Verification items for the finished model (mm, model axes). Give positions to 0.01 mm unless a question says otherwise; leave off trailing zeros. Order: outer loops, then holes, each group sorted by start corner. A loop starts at its lowest first (then second) coordinate and runs counter-clockwise, first axis right, second up.
(1) Sectioned sample at B-B on x = 30. Record the cut outline in (y, z), plus the area to 3 significant figures.
(2) Scan lines: L1, parallel to X at y = -48.5, z = 2.75; L2, parallel to X at y = 82, z = 0.8; L3, parallel to Y at x = 93, z = 2.6. Record each from-to range of solid material in increasing order.
(3) Sectioned sample at A-A on y = 37. Record the cut outline in (x, z), plus the area to 3 significant figures.
(4) Gauge pin test, flat ends, axial feed: pin 1 (0.9 mm diameter, centred on x = 106, z = 1, fed in from +Y); pin 2 (0.9 mm diameter, centred on y = -102, z = 1, fed in from -X); pin 3 (0.9 mm diameter, centred on x = -106.5, z = 1, fed in from -Y). Record the tip position at first contact, or that the pin passes through.
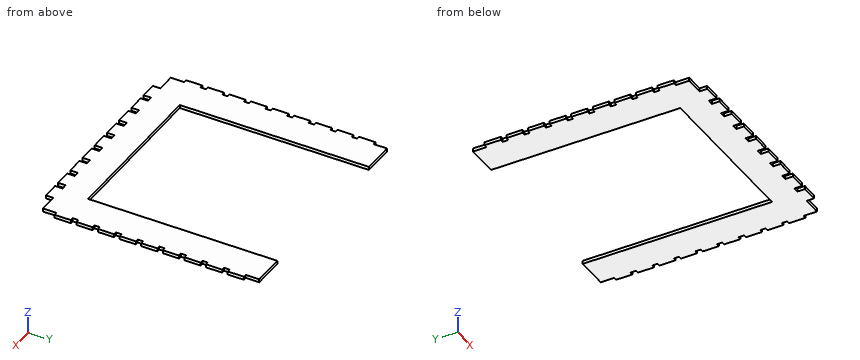
```python
from build123d import *

# Parameters (mm, degrees)
BOSS_EXTRUDE1_DEPTH = 3


with BuildPart() as part:
    # Sketch1 → Boss-Extrude1 (new body)
    with BuildSketch(Plane.XY):
        Polygon((-75, 100), (-104.5, 100), (-104.5, 87.5), (-107.5, 87.5), (-107.5, 72.5), (-104.5, 72.5), (-104.5, 67.5), (-107.5, 67.5), (-107.5, 52.5), (-104.5, 52.5), (-104.5, 47.5), (-107.5, 47.5), (-107.5, 32.5), (-104.5, 32.5), (-104.5, 27.5), (-107.5, 27.5), (-107.5, 12.5), (-104.5, 12.5), (-104.5, 7.5), (-107.5, 7.5), (-107.5, -7.5), (-104.5, -7.5), (-104.5, -12.5), (-107.5, -12.5), (-107.5, -27.5), (-104.5, -27.5), (-104.5, -32.5), (-107.5, -32.5), (-107.5, -47.5), (-104.5, -47.5), (-104.5, -52.5), (-107.5, -52.5), (-107.5, -67.5), (-104.5, -67.5), (-104.5, -72.5), (-107.5, -72.5), (-107.5, -87.5), (-104.5, -87.5), (-104.5, -100), (-87.5, -100), (-87.5, -107), (-72.5, -107), (-72.5, -100), (-67.5, -100), (-67.5, -107), (-52.5, -107), (-52.5, -100), (-47.5, -100), (-47.5, -107), (-32.5, -107), (-32.5, -100), (-27.5, -100), (-27.5, -107), (-12.5, -107), (-12.5, -100), (-7.5, -100), (-7.5, -107), (7.5, -107), (7.5, -100), (12.5, -100), (12.5, -107), (27.5, -107), (27.5, -100), (32.5, -100), (32.5, -107), (47.5, -107), (47.5, -100), (52.5, -100), (52.5, -107), (67.5, -107), (67.5, -100), (72.5, -100), (72.5, -107), (87.5, -107), (87.5, -100), (104.5, -100), (104.5, -87.5), (107.5, -87.5), (107.5, -72.5), (104.5, -72.5), (104.5, -67.5), (107.5, -67.5), (107.5, -52.5), (104.5, -52.5), (104.5, -47.5), (107.5, -47.5), (107.5, -32.5), (104.5, -32.5), (104.5, -27.5), (107.5, -27.5), (107.5, -12.5), (104.5, -12.5), (104.5, -7.5), (107.5, -7.5), (107.5, 7.5), (104.5, 7.5), (104.5, 12.5), (107.5, 12.5), (107.5, 27.5), (104.5, 27.5), (104.5, 32.5), (107.5, 32.5), (107.5, 47.5), (104.5, 47.5), (104.5, 52.5), (107.5, 52.5), (107.5, 67.5), (104.5, 67.5), (104.5, 72.5), (107.5, 72.5), (107.5, 87.5), (104.5, 87.5), (104.5, 100), (75, 100), (75, -75), (-75, -75), align=None)
    extrude(amount=BOSS_EXTRUDE1_DEPTH)


solid = part.part
```
Ans:
1. outline: (-100, 0) - (-75, 0) - (-75, 3) - (-100, 3) - close
1. area: 75.0 mm2
2. L1: x = -104.5 to -75, 75 to 104.5
2. L2: x = -107.5 to -75, 75 to 107.5
2. L3: y = -100 to 100
3. outline: (-107.5, 0) - (-75, 0) - (-75, 3) - (-107.5, 3) - close; (75, 0) - (107.5, 0) - (107.5, 3) - (75, 3) - close
3. area: 195 mm2
4. pin 1: stops at y = 87.5
4. pin 2: stops at x = -87.5
4. pin 3: stops at y = -87.5
